from build123d import *

# Parameters (mm, degrees)
SKETCH_2_R          = 1.6
EXTRUDE_1_DEPTH     = 3
FILLET_1_R          = 3
FILLET_2_R          = 2
FILLET_3_R          = 3
SKETCH_4_W          = 20
SKETCH_4_H          = 8
CUT_EXTRUDE_2_DEPTH = 77.136305652
FILLET_5_R          = 2
SKETCH_5_R          = 1.6
CUT_EXTRUDE_3_DEPTH = 77.136305652


with BuildPart() as part:
    # 草图2 → 凸台-拉伸1 (new body)
    with BuildSketch(Plane.XY):
        Polygon((-22.933897075, 18), (-47.5, -60), (-39.5, -60), (-10, -4), (10, -4), (39.5, -60), (47.5, -60), (22.933897075, 18), align=None)
        with Locations((-20, 14)):
            Circle(SKETCH_2_R, mode=Mode.SUBTRACT)
        with Locations((20, 14)):
            Circle(SKETCH_2_R, mode=Mode.SUBTRACT)
    extrude(amount=EXTRUDE_1_DEPTH)

    # 圆角1
    fillet_1_edges = [part.edges().sort_by_distance(p)[0] for p in [
        (22.933897075, 18, 1.5),
        (-22.933897075, 18, 1.5),
    ]]
    fillet(fillet_1_edges, radius=FILLET_1_R)

    # 圆角2
    fillet_2_edges = [part.edges().sort_by_distance(p)[0] for p in [
        (47.5, -60, 1.5),
        (39.5, -60, 1.5),
        (-39.5, -60, 1.5),
        (-47.5, -60, 1.5),
    ]]
    fillet(fillet_2_edges, radius=FILLET_2_R)

    # 圆角3
    fillet_3_edges = [part.edges().sort_by_distance(p)[0] for p in [
        (10, -4, 1.5),
        (-10, -4, 1.5),
    ]]
    fillet(fillet_3_edges, radius=FILLET_3_R)

    # 草图4 → 切除-拉伸2 (cut, through all)
    with BuildSketch(Plane.XY.offset(3)):
        with Locations((0, 6.8)):
            Rectangle(SKETCH_4_W, SKETCH_4_H)
    extrude(amount=-CUT_EXTRUDE_2_DEPTH, mode=Mode.SUBTRACT)

    # 圆角5
    fillet_5_edges = [part.edges().sort_by_distance(p)[0] for p in [
        (-10, 2.8, 1.5),
        (-10, 10.8, 1.5),
        (10, 10.8, 1.5),
        (10, 2.8, 1.5),
    ]]
    fillet(fillet_5_edges, radius=FILLET_5_R)

    # 草图5 → 切除-拉伸3 (cut, through all)
    with BuildSketch(Plane.XY.offset(3)):
        with Locations((-25, -11)):
            Circle(SKETCH_5_R)
        with Locations((25, -11)):
            Circle(SKETCH_5_R)
    extrude(amount=-CUT_EXTRUDE_3_DEPTH, mode=Mode.SUBTRACT)


solid = part.part
Geometry: final body of the model. Coordinates: model frame, mm. A direction names the side the tool comes from. Round coordinates to 2 decimals unless told otherwise and drop trailing zeros. Loops run counter-clockwise (first coordinate to the right, second up) from the corner with the lowest first, then second, coordinate; pieces in that order, holes last. Notation, with made-up numbers: M 46.5,-37.5 L 91.5,-37.5 A32 ccw 91.5,-3.5 Z; hole C -2,46 d9. An arc over 180 degrees is marked long. One line per question, with ' | ' between items.
(1) Access query for faces 1 (the flat face through (0, -4, 1)), 2 (the cylindrical face through (9.43, 10.2, 1.48)), 3 (the flat face through (3, -1, 3)). Directions: +Z, -Z, +X, -X, +Y, -Y. A direction counts if a zero-diameter tool reaches every point of the face in a straight line with its end or side. Return the directions, or none.
Check result:
face 1: +Z, -Z, -Y | face 2: +Z, -Z | face 3: +Z, +X, -X, +Y, -Y
(2) Cut plane A-A on z = 0.9. Return the cut outline in (x, y).
Check result:
outline: M -46.68,-57.4 A2 ccw -44.77,-60 L -40.71,-60 A2 ccw -38.94,-58.93 L -10.84,-5.6 A3 cw -8.19,-4 L 8.19,-4 A3 cw 10.84,-5.6 L 38.94,-58.93 A2 ccw 40.71,-60 L 44.77,-60 A2 ccw 46.68,-57.4 L 23.59,15.9 A3 ccw 20.73,18 L -20.73,18 A3 ccw -23.59,15.9 Z; hole C -25,-11 d3.2; hole C -20,14 d3.2; hole M -10,4.8 A2 ccw -8,2.8 L 8,2.8 A2 ccw 10,4.8 L 10,8.8 A2 ccw 8,10.8 L -8,10.8 A2 ccw -10,8.8 Z; hole C 20,14 d3.2; hole C 25,-11 d3.2
(3) Pull-direction query (X, two-part tool) for faces 4 (the flat face through (-10, 7, 2)), 5 (the flat face through (0, 18, 1)), 6 (the cylindrical face through (22.49, 17.43, 1.52)); classes: +X half, -X half, draft (parallel to the pull), parting line (faces both ways), or undercut.
Check result:
face 4: undercut | face 5: draft | face 6: +X half
(4) Cut plane D-D on y = 14. Return the cut outline in (x, z), plus the area to 3 significant figures.
Check result:
outline: M -24.19,0 L -21.6,0 L -21.6,3 L -24.19,3 Z; M -18.4,0 L 18.4,0 L 18.4,3 L -18.4,3 Z; M 21.6,0 L 24.19,0 L 24.19,3 L 21.6,3 Z | area: 126 mm2
(5) Cut plane C-C on x = -25. Return the cut outline in (y, z).
Check result:
outline: M -32.47,0 L -12.6,0 L -12.6,3 L -32.47,3 Z; M -9.4,0 L 11.44,0 L 11.44,3 L -9.4,3 Z
(6) Material intervals for line 1 along Y through (x, z) = (6.5, 1.8); line 2 along X through (y, z) = (8, 0.45); line 3 along X through (y, z) = (-39.5, 1.8), sorted ascending. Write a range as from..to.
Check result:
line 1: y = -4..2.8, 10.8..18 | line 2: x = -26.08..-10, 10..26.08 | line 3: x = -41.04..-28.7, 28.7..41.04
(7) Cut plane B-B on y = -46.5. Return the cut outline in (x, z).
Check result:
outline: M -43.25,0 L -32.39,0 L -32.39,3 L -43.25,3 Z; M 32.39,0 L 43.25,0 L 43.25,3 L 32.39,3 Z
(8) Contact query for flat-ended pins moving along their axis: P1, Ø2.5, axis at x = -25, y = -11, coming from the +Z side; P2, Ø1, axis at y = -16.5, z = 2.5, coming from the +X side. Output: stop coordinate, or through.
Check result:
P1: passes through | P2: stops at x = 33.96
